Autodesk Inventor part; units mm, degrees
ref_plane "YZ Plane" through (0, 0, 0) normal (1, 0, 0) x (0, 1, 0)
ref_plane "XZ Plane" through (0, 0, 0) normal (0, 1, 0) x (-1, 0, 0)
ref_plane "XY Plane" through (0, 0, 0) normal (0, 0, 1) x (1, 0, 0)
sketch "Эскиз1" plane through (0, 0, 0) normal (0, 0, 1) x (1, 0, 0)
  line L0 (0, 0) -> (20, 0)
  line L1 (20, 0) -> (20, 30)
  line L2 (20, 30) -> (0, 30)
  line L3 (0, 30) -> (0, 0)
  dimension "d0" = 20
  dimension "d1" = 30
revolve "Вращение1" add sketch "Эскиз1" angle 360 about axis through (0, 0, 0) along (1, 0, 0)
sketch "Эскиз2" plane through (0, 0, 0) normal (0, 0, 1) x (1, 0, 0)
  line L0 (0, -30) -> (0, 30) construction
  line L1 (0, 20.647) -> (0, 23.353)
  line L2 (0, 23.353) -> (4, 24.5)
  line L3 (4, 24.5) -> (4, 19.5)
  line L4 (4, 19.5) -> (0, 20.647)
  line L5 (4, 22) -> (0, 22) construction
  line L6 (0, 0) -> (20.0289, 0)
  dimension "d3" = 74
  dimension "d4" = 74
  dimension "d5" = 5
  dimension "d6" = 4
  dimension "d7" = 22
revolve "Вращение2" cut sketch "Эскиз2" angle 360 about axis through (0, 0, 0) along (1, 0, 0)
sketch "Эскиз3" plane through (0, 0, 0) normal (-1, 0, 0) x (0, 0, 1)
  line L0 (-30, -26.5) -> (-30, 26.5)
  line L1 (-30, 26.5) -> (30, 26.5)
  line L2 (30, 26.5) -> (30, -26.5)
  line L3 (30, -26.5) -> (-30, -26.5)
  point P0 (0, 0)
  point P1 (-30, 0)
  point P2 (30, 0)
  point P3 (0, 26.5)
  dimension "d9" = 53
  dimension "d10" = 60
extrude "Выдавливание1" cut sketch "Эскиз3" against normal blind 20 keep common part
properties part number "711117"
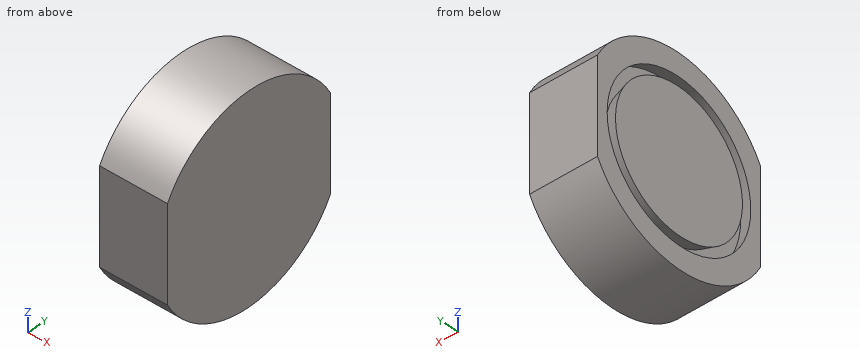
Build history of the part. All positions in model axes, mm. Give positions to 0.01 mm unless a question says otherwise; leave off trailing zeros. Write each loop counter-clockwise with the first axis right and the second up, starting at its lowest first coordinate (ties: lowest second). Pieces come first, ordered by that corner, then holes. Notation, with made-up numbers: (21.25, -29.5) - (52.25, -29.5) arc R34 cw to (52.25, 9.5) - close; hole circle Ø2 at (-15, 34). An arc over 180 degrees is marked (long way). Use one line per item in the form item = value. Start each with the question number.
1. Probe line 1 (Z direction, x = 2, y = 10.5); line 2 (Z direction, x = 3.5, y = 3); line 3 (Y direction, x = 3.25, z = 4). List the from-to ranges inside material, lowest first. Write a range as [from, to].
2. Band-saw the part on A-A on y = 0. Write the cut outline in (x, z), plus the area to 3 significant figures.
3. Drop flat-ended pins along their axis: pin 1 Ø6 at (x, y) = (3.5, -13.5) entering from +Z; pin 2 Ø1 at (x, y) = (15, 12) entering from -Z; pin 3 Ø4 at (x, y) = (7, -9.5) entering from -Z. Give the stop position or say it passes through.
4. Band-saw the part on B-B on z = 0. Write the cut outline in (x, y), plus the area to 3 significant figures.
5. Band-saw the part on C-C on x = 8. Write the cut outline in (y, z), plus the area to 3 significant figures.
Conclusion:
q1.line_1 = [-28.1, -21.5], [-17.11, 17.11], [21.5, 28.1]
q1.line_2 = [-29.85, -24.17], [-19.41, 19.41], [24.17, 29.85]
q1.line_3 = [-26.5, -23.95], [-19.31, 19.31], [23.95, 26.5]
q2.outline = (0, -30) - (20, -30) - (20, 30) - (0, 30) - (0, 23.35) - (4, 24.5) - (4, 19.5) - (0, 20.65) - (0, -20.65) - (4, -19.5) - (4, -24.5) - (0, -23.35) - close
q2.area = 1,170 mm²
q3.pin_1 = 28.1
q3.pin_2 = -27.71
q3.pin_3 = -29.05
q4.outline = (0, -26.5) - (20, -26.5) - (20, 26.5) - (0, 26.5) - (0, 23.35) - (4, 24.5) - (4, 19.5) - (0, 20.65) - (0, -20.65) - (4, -19.5) - (4, -24.5) - (0, -23.35) - close
q4.area = 1,030 mm²
q5.outline = (-26.5, -14.06) arc R30 ccw to (26.5, -14.06) - (26.5, 14.06) arc R30 ccw to (-26.5, 14.06) - close
q5.area = 2,690 mm²
